from build123d import *

# Parameters (mm, degrees)
SKETCH1_R             = 0.4
BOSS_EXTRUDE1_DEPTH   = 3.5
BOSS_EXTRUDE1_2_DEPTH = 3.5
BOSS_EXTRUDE1_3_DEPTH = 3.5
BOSS_EXTRUDE1_4_DEPTH = 3.5
BOSS_EXTRUDE1_5_DEPTH = 3.5
SKETCH1_W             = 1
SKETCH1_H             = 1.8
BOSS_EXTRUDE1_6_DEPTH = 3.5
BOSS_EXTRUDE1_7_DEPTH = 3.5
SKETCH2_W             = 12.4
SKETCH2_H             = 13.2
BOSS_EXTRUDE2_DEPTH   = 6
SKETCH3_W             = 12.4
SKETCH3_H             = 15.3
BOSS_EXTRUDE3_DEPTH   = 0.5
SKETCH4_R             = 3
BOSS_EXTRUDE4_DEPTH   = 24
CUT_EXTRUDE1_DEPTH    = 12


with BuildPart() as part:
    # Sketch1 → Boss-Extrude1 (new body)
    with BuildSketch(Plane(origin=(0, 0, 0), x_dir=(1, 0, 0), z_dir=(0, 1, 0))):
        with Locations((-2.5, -7.5)):
            Circle(SKETCH1_R)
    extrude(amount=-BOSS_EXTRUDE1_DEPTH)



with BuildPart() as body_2:
    # Sketch1 → Boss-Extrude1 2 (new body)
    with BuildSketch(Plane(origin=(0, 0, 0), x_dir=(1, 0, 0), z_dir=(0, 1, 0))):
        with Locations((0, -7.5)):
            Circle(SKETCH1_R)
    extrude(amount=-BOSS_EXTRUDE1_2_DEPTH)


with BuildPart() as body_3:
    # Sketch1 → Boss-Extrude1 3 (new body)
    with BuildSketch(Plane(origin=(0, 0, 0), x_dir=(1, 0, 0), z_dir=(0, 1, 0))):
        with Locations((2.5, -7.5)):
            Circle(SKETCH1_R)
    extrude(amount=-BOSS_EXTRUDE1_3_DEPTH)


with BuildPart() as body_4:
    # Sketch1 → Boss-Extrude1 4 (new body)
    with BuildSketch(Plane(origin=(0, 0, 0), x_dir=(1, 0, 0), z_dir=(0, 1, 0))):
        with Locations((2.5, 7)):
            Circle(SKETCH1_R)
    extrude(amount=-BOSS_EXTRUDE1_4_DEPTH)


with BuildPart() as body_5:
    # Sketch1 → Boss-Extrude1 5 (new body)
    with BuildSketch(Plane(origin=(0, 0, 0), x_dir=(1, 0, 0), z_dir=(0, 1, 0))):
        with Locations((-2.5, 7)):
            Circle(SKETCH1_R)
    extrude(amount=-BOSS_EXTRUDE1_5_DEPTH)


with BuildPart() as body_6:
    # Sketch1 → Boss-Extrude1 6 (new body)
    with BuildSketch(Plane(origin=(0, 0, 0), x_dir=(1, 0, 0), z_dir=(0, 1, 0))):
        with Locations((-5.6, 0)):
            Rectangle(SKETCH1_W, SKETCH1_H)
    extrude(amount=-BOSS_EXTRUDE1_6_DEPTH)



with BuildPart() as body_7:
    # Sketch1 → Boss-Extrude1 7 (new body)
    with BuildSketch(Plane(origin=(0, 0, 0), x_dir=(1, 0, 0), z_dir=(0, 1, 0))):
        with Locations((5.6, 0)):
            Rectangle(SKETCH1_W, SKETCH1_H)
    extrude(amount=-BOSS_EXTRUDE1_7_DEPTH)


with BuildPart() as body_6_1:
    add(body_6.part)

    add(body_7.part)  # Boss-Extrude2 merges body 7
    # Sketch2 → Boss-Extrude2 (add)
    with BuildSketch(Plane(origin=(0, 0, 0), x_dir=(1, 0, 0), z_dir=(0, 1, 0))):
        Rectangle(SKETCH2_W, SKETCH2_H)
    extrude(amount=BOSS_EXTRUDE2_DEPTH)


with BuildPart() as part_1:
    add(part.part)

    add(body_2.part)  # Boss-Extrude3 merges body 2

    add(body_3.part)  # Boss-Extrude3 merges body 3

    add(body_4.part)  # Boss-Extrude3 merges body 4

    add(body_5.part)  # Boss-Extrude3 merges body 5

    add(body_6_1.part)  # Boss-Extrude3 merges body 6
    # Sketch3 → Boss-Extrude3 (add)
    with BuildSketch(Plane(origin=(0, 0, 0), x_dir=(1, 0, 0), z_dir=(0, 1, 0))):
        with Locations((0, -0.25)):
            Rectangle(SKETCH3_W, SKETCH3_H)
    extrude(amount=BOSS_EXTRUDE3_DEPTH)

    # Sketch4 → Boss-Extrude4 (add)
    with BuildSketch(Plane(origin=(0, 6, 0), x_dir=(1, 0, 0), z_dir=(0, 1, 0))):
        Circle(SKETCH4_R)
    extrude(amount=BOSS_EXTRUDE4_DEPTH)

    # Sketch5 → Cut-Extrude1 (cut)
    with BuildSketch(Plane(origin=(0, 30, 0), x_dir=(1, 0, 0), z_dir=(0, 1, 0))):
        with BuildLine():
            Line((-2.598076211, -1.5), (2.598076211, -1.5))
            ThreePointArc((2.598076211, -1.5), (0, -3), (-2.598076211, -1.5))
        make_face()
    extrude(amount=-CUT_EXTRUDE1_DEPTH, mode=Mode.SUBTRACT)


solid = part_1.part
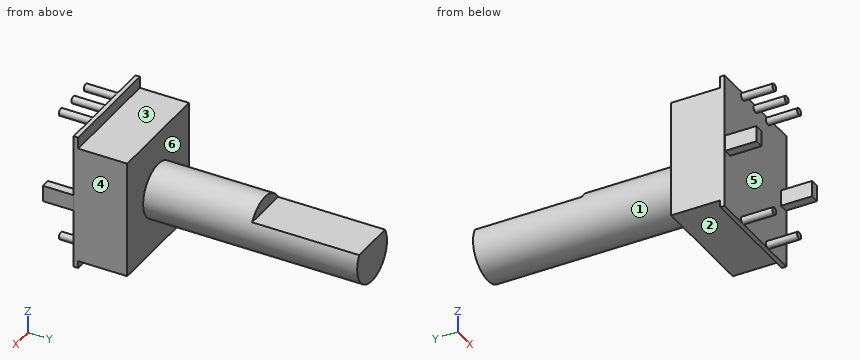
The listing builds one solid part. Answer for the finished solid, in the listing's coordinates (mm). Face numbers are marked on the shaded views. A direction names the side the tool comes from. Coordinates: 2 decimals unless noted, no trailing zeros. Write each loop counter-clockwise with the first axis right and the second up, starting at its lowest first coordinate (ties: lowest second). Pieces come first, ordered by that corner, then holes. Notation, with made-up numbers: (73.25, -16) -> (119.25, -16) arc R25 ccw to (119.25, -1) -> close; hole circle Ø3 at (-9, 23.5). An arc over 180 degrees is marked (long way). One line per question, with ' | ' between items.
1. Given pin 1 Ø1 at (x, z) = (3, -1) entering from -Y; pin 2 Ø1.6 at (x, y) = (2.5, 3.5) entering from +Z; pin 3 Ø2 at (y, z) = (-2, 0) entering from +X, each flat-ended and moving along its own axis, determine where each tip first touches the part or whether it passes through.
Verdict:
pin 1: stops at y = 0 | pin 2: stops at z = 6.6 | pin 3: stops at x = 6.1
2. Section A-A (y = -1) is taken. Determine the outline of the cut face in (x, z), and give its area (3 significant figures).
Verdict:
outline: (-6.1, -0.9) -> (-5.1, -0.9) -> (-5.1, 0.9) -> (-6.1, 0.9) -> close; circle Ø0.8 at (-2.5, -7); circle Ø0.8 at (-2.5, 7.5); circle Ø0.8 at (0, 7.5); circle Ø0.8 at (2.5, -7); circle Ø0.8 at (2.5, 7.5); (5.1, -0.9) -> (6.1, -0.9) -> (6.1, 0.9) -> (5.1, 0.9) -> close | area: 6.11 mm^2
3. Which of the six approach directions +Z, -Z, +X, -X, +Y, -Y give full straight-line access (tool end or side, diameter ignored) to the marked faces 1, 2 and 3?
Verdict:
face 1: +Y | face 2: -Z, +X, -X, +Y | face 3: +Z, +X, -X, +Y
4. Section B-B (z = 0) is taken. Determine the outline of the cut face in (x, y), and give its area (3 significant figures).
Verdict:
outline: (-6.2, 0) -> (-6.1, 0) -> (-6.1, -3.5) -> (-5.1, -3.5) -> (-5.1, 0) -> (5.1, 0) -> (5.1, -3.5) -> (6.1, -3.5) -> (6.1, 0) -> (6.2, 0) -> (6.2, 6) -> (3, 6) -> (3, 30) -> (-3, 30) -> (-3, 6) -> (-6.2, 6) -> close | area: 225 mm^2
5. Section C-C (x = 1.5) is taken. Determine the outline of the cut face in (y, z), and give its area (3 significant figures).
Verdict:
outline: (0, -7.4) -> (0.5, -7.4) -> (0.5, -6.6) -> (6, -6.6) -> (6, -2.6) -> (30, -2.6) -> (30, 1.5) -> (18, 1.5) -> (18, 2.6) -> (6, 2.6) -> (6, 6.6) -> (0.5, 6.6) -> (0.5, 7.9) -> (0, 7.9) -> close | area: 192 mm^2
6. For a pull along X with two mould halves and no side action, classify the marked faces 4, 5 and 6 as released by +X, released by -X, zero draft, split by the parting line, or undercut.
Verdict:
face 4: released by +X | face 5: undercut | face 6: zero draft
7. Straight lines are drawn through the part: line 1 (Y direction, x = -0.75, z = -6); line 2 (X direction, y = 9, z = 1.5); line 3 (Z direction, x = 0.75, y = 3.5). For each, find the intervals that lie inside material, in ascending order.
Verdict:
line 1: y = 0 to 6 | line 2: x = -2.6 to 2.6 | line 3: z = -6.6 to 6.6
8. Section D-D (z = 7.5) is taken. Determine the outline of the cut face in (x, y).
Verdict:
outline: (-6.2, 0) -> (-2.9, 0) -> (-2.9, -3.5) -> (-2.1, -3.5) -> (-2.1, 0) -> (-0.4, 0) -> (-0.4, -3.5) -> (0.4, -3.5) -> (0.4, 0) -> (2.1, 0) -> (2.1, -3.5) -> (2.9, -3.5) -> (2.9, 0) -> (6.2, 0) -> (6.2, 0.5) -> (-6.2, 0.5) -> close
